For this review, take the finished solid that the model builds, in its own axes (mm). Face numbers are marked on the shaded views. A direction names the side the tool comes from. Coordinates: 2 decimals unless noted, no trailing zeros. Write each loop counter-clockwise with the first axis right and the second up, starting at its lowest first coordinate (ties: lowest second). Pieces come first, ordered by that corner, then holes. Notation, with made-up numbers: (-39.5, 29.25) -> (11.5, 29.25) arc R20 cw to (11.5, 63.25) -> close; hole circle Ø4 at (60.25, -11). An arc over 180 degrees is marked (long way). Put each result on its own line as item: value. Start each with the question number.
Item 1: Consider section B-B on y = -27.5. Give the boundary of the cut face in (x, z), and give its area (3 significant figures).
Item 2: To check wall thickness, follow L1, parallel to Y at x = 0.85, z = 0; L2, parallel to Z at x = -0.75, y = -27.5; L3, parallel to Z at x = -0.85, y = 27.5. State the ranges of each line that lie inside material, in increasing order.
Item 3: Consider section A-A on z = 0. Give the boundary of the cut face in (x, y).
Item 4: For the marked faces 5, 6 and 7, list the 3-axis set-ups (+Z, -Z, +X, -X, +Y, -Y) from which the entire face can be reached by the end or side of a thin tool; tool diameter is ignored.
Item 5: Insertion check: P1, Ø1, axis at x = 1, y = -4, coming from the +Z side; P2, Ø1, axis at x = 4.5, z = 1.5, coming from the +Y side; P3, Ø2, axis at y = 27.5, z = 0.5, coming from the +X side. Each pin has a flat end and moves straight along its axis. Give the tip position at first contact, or say it passes through.
Item 6: Consider section C-C on x = 3.25. Give the boundary of the cut face in (y, z).
Item 7: The part is to be moulded in two halves that separate along Y. For the marked faces 1, 2, 3 and 4, say which applies: +Y half, -Y half, draft (parallel to the pull), parting line (faces both ways), or undercut.
Item 8: Consider section D-D on x = -0.75. Give the boundary of the cut face in (y, z), and give its area (3 significant figures).
Autodesk Inventor part; units mm, degrees
ref_plane "YZ Plane" through (0, 0, 0) normal (1, 0, 0) x (0, 1, 0)
ref_plane "XZ Plane" through (0, 0, 0) normal (0, 1, 0) x (-1, 0, 0)
ref_plane "XY Plane" through (0, 0, 0) normal (0, 0, 1) x (1, 0, 0)
sketch "Sketch1" plane through (0, 0, 0) normal (1, 0, 0) x (0, 1, 0)
  line L0 (-42.7, 0) -> (42.7, 0)
  line L1 (0, -4.2) -> (0, 4.2)
  circle A0 centre (-27.5, 0) radius 1.25
  circle A1 centre (-27.5, 0) radius 3
  circle A2 centre (27.5, 0) radius 3 construction
  line L2 (-27.5, 3) -> (27.5, 3)
  line L3 (-27.5, -3) -> (27.5, -3)
  line L4 (27.5, 3) -> (27.5, -3) construction
  line L5 (27.5, 2) -> (27.5, -2) construction
  arc A3 (27.5, -3) -> (27.5, 3) centre (27.5, 0) ccw
  circle A4 centre (-27.5, 0) radius 2.2678 construction
  circle A5 centre (27.5, 0) radius 1
  point P0 (0, 0)
  dimension "d4" = 6
  dimension "d7" = 55
  dimension "d8" = 2.5
  dimension "d10" = 0
  dimension "d30" = 2
extrude "ext_main" add sketch "Sketch1" along normal mid plane 3.5 contours A0 L0 A1 | L0 A1 A0 | A1 L2 L1 L0 | L0 L1 L3 A1 | L1 L2 A3 L0 A5 | L0 A5 A3 L3 L1
sketch "Sketch3" plane through (0, 0, 0) normal (1, 0, 0) x (0, 1, 0)
  arc A0 (-27.5, 3) -> (-27.5, -3) centre (-27.5, 0) ccw
  circle A1 centre (-27.5, 0) radius 1.25
  arc A2 (27.5, -3) -> (27.5, 3) centre (27.5, 0) ccw
  circle A3 centre (-27.5, 0) radius 3 construction
  circle A4 centre (27.5, 0) radius 3 construction
  line L0 (-25.2639, 2) -> (25.2639, 2) construction
  line L1 (-42.7, 0) -> (42.7, 0)
  line L2 (0, -4.2579) -> (0, 4.2579)
  line L3 (27.5, 3) -> (-27.5, 3)
  line L4 (24.1192, 2) -> (26.5141, 2.8334)
  arc A5 (27.5, 3) -> (26.5141, 2.8334) centre (27.5, 0) ccw
  line L5 (-24.3389, 2) -> (24.1192, 2)
  circle A6 centre (-27.5, 0) radius 2.75
  line L6 (-24.3389, 2) -> (-26.7882, 2.6563)
  arc A7 (26.5141, -2.8334) -> (27.5, -3) centre (27.5, 0) ccw
  line L7 (24.1192, -2) -> (-25.2639, -2) construction
  line L8 (-24.3389, -2) -> (-26.7882, -2.6563)
  line L9 (24.1192, -2) -> (-24.3389, -2)
  line L10 (24.1192, -2) -> (26.5141, -2.8334)
  point P0 (0, 0)
  dimension "d16" = 1
  dimension "d21" = 5.5
  dimension "d22" = 15
extrude "ext_cutaway" cut sketch "Sketch3" along normal through all both and the other way through all contours A6 L1 A1 | L1 A1 A6 | L5 L4 A5 A2 L1 L2 | L2 L1 A6 L6 L5 | A6 L1 L2 L9 L8 | L1 A2 A7 L10 L9 L2 keep common part
sketch "Sketch4" plane through (1.75, 0, 0) normal (1, 0, 0) x (0, 0, -1)
  arc A0 (2.8334, 26.5141) -> (-2.8334, 26.5141) centre (0, 27.5) ccw
  circle A1 centre (0, 27.5) radius 1
  circle A2 centre (0, 27.5) radius 3
  line L0 (-4.2, 0) -> (4.2, 0)
  line L1 (-3, 27.5) -> (3, 27.5) construction
  circle A3 centre (0, 27.5) radius 2 construction
  arc A4 (-1.4283, 28.9) -> (-1.4283, 26.1) centre (0, 27.5) ccw
  arc A5 (1.4283, 26.1) -> (1.4283, 28.9) centre (0, 27.5) ccw
  line L2 (-1.4283, 28.9) -> (1.4283, 28.9)
  line L3 (-1.4283, 26.1) -> (1.4283, 26.1)
  point P0 (0, 0)
  dimension "d23" = 4
  dimension "d25" = 2.8
extrude "ext_potshaft" add sketch "Sketch4" along normal blind 3.5 contours A2 A0
extrude "ext_cut_potshaft" cut sketch "Sketch4" against normal blind 1 contours L2 A5 L3 A4
equation "\"d8\" = screw_m2_bore_loose"
equation "\"d30\" = screw_m2_bore_selfthreading"
equation "\"d21\" = general_bore_smallersupport_diameter"
properties part number "empty"
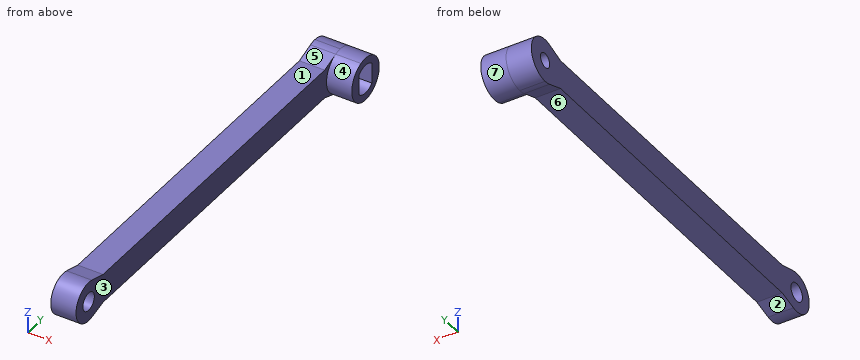
Return value:
1. outline: (-1.75, -2.75) -> (1.75, -2.75) -> (1.75, -1.25) -> (-1.75, -1.25) -> close; (-1.75, 1.25) -> (1.75, 1.25) -> (1.75, 2.75) -> (-1.75, 2.75) -> close
1. area: 10.5 mm^2
2. L1: -30.25 to -28.75, -26.25 to 26.1, 28.9 to 30.5
2. L2: -2.75 to -1.25, 1.25 to 2.75
2. L3: -3 to -1, 1 to 3
3. outline: (-1.75, -30.25) -> (1.75, -30.25) -> (1.75, -28.75) -> (-1.75, -28.75) -> close; (-1.75, -26.25) -> (1.75, -26.25) -> (1.75, 24.5) -> (5.25, 24.5) -> (5.25, 26.1) -> (0.75, 26.1) -> (0.75, 26.5) -> (-1.75, 26.5) -> close; (-1.75, 28.5) -> (0.75, 28.5) -> (0.75, 28.9) -> (5.25, 28.9) -> (5.25, 30.5) -> (-1.75, 30.5) -> close
4. face 5: +Z, +X, -X
4. face 6: -Z, +X, -X
4. face 7: +X, -X
5. P1: z = 2
5. P2: y = 30.33
5. P3: x = 0.75
6. outline: circle Ø6 at (27.5, 0); hole (26.1, -1.43) arc R2 ccw to (28.9, -1.43) -> (28.9, 1.43) arc R2 ccw to (26.1, 1.43) -> close
7. face 1: undercut
7. face 2: undercut
7. face 3: draft
7. face 4: -Y half
8. outline: (-26.79, -2.66) -> (-24.34, -2) -> (24.12, -2) -> (26.51, -2.83) arc R3 ccw to (27.5, -3) arc R3 ccw to (27.5, 3) arc R3 ccw to (26.51, 2.83) -> (24.12, 2) -> (-24.34, 2) -> (-26.79, 2.66) arc R2.75 ccw (long way) to start; hole circle Ø2.5 at (-27.5, 0); hole circle Ø2 at (27.5, 0)
8. area: 244 mm^2
